Could you check a few things on this model? Use its own coordinates, in mm. A direction names the side the tool comes from. Give positions to 0.01 mm unless a question says otherwise; leave off trailing zeros. Write each loop counter-clockwise with the first axis right and the second up, starting at its lowest first coordinate (ties: lowest second). Pieces come first, ordered by that corner, then holes. Notation, with made-up numbers: (31.25, 20.25) - (44.25, 20.25) arc R27 cw to (44.25, 39.25) - close; hole circle Ø1 at (57.5, 69). An arc over 180 degrees is marked (long way). Answer in a Markdown table with one row per item.
from build123d import *

# Parameters (mm, degrees)
ESQUISSE1_W        = 155
ESQUISSE1_H        = 34
BOSS_EXTRU_1_DEPTH = 49
ESQUISSE2_R        = 2
BOSS_EXTRU_2_DEPTH = 5


with BuildPart() as part:
    # Esquisse1 → Boss.-Extru.1 (new body)
    with BuildSketch(Plane(origin=(0, 0, 0), x_dir=(1, 0, 0), z_dir=(0, 1, 0))):
        with Locations((77.5, 17)):
            Rectangle(ESQUISSE1_W, ESQUISSE1_H)
    extrude(amount=BOSS_EXTRU_1_DEPTH)

    # Esquisse2 → Boss.-Extru.2 (add)
    with BuildSketch(Plane(origin=(155, 0, 0), x_dir=(0, 0, -1), z_dir=(1, 0, 0))):
        with Locations(Location((14.5, 46, 0), (0, 0, 180))):
            Circle(ESQUISSE2_R)
        with Locations(Location((19.5, 46, 0), (0, 0, 180))):
            Circle(ESQUISSE2_R)
    extrude(amount=BOSS_EXTRU_2_DEPTH)


solid = part.part
1) Will this pin go through, and if not, where does the flat tip stop? P1, Ø8, axis at y = 39.5, z = -8, coming from the +X side.
Check values:
| item | result |
|---|---|
| P1 | stops at x = 155 |
2) If I drill on line 1 (X direction, y = 36, z = -13.5), over which ranges is the centre line in solid material (lowest first)?
Check values:
| item | result |
|---|---|
| line 1 | x = 0 to 155 |
3) On a 3-axis mill with a long thin cutter (end or side, diameter ignored), from which of +Z, -Z, +X, -X, +Y, -Y can I reach the whole of each face in a straight line? I mean faces 5 (the face through (0, 24, -17)), 6 (the face through (157.465, 47.952, -14.934)). Say none if no direction works.
Check values:
| item | result |
|---|---|
| face 5 | +Z, -Z, -X, +Y, -Y |
| face 6 | +X |
4) Imagine slicing it at C-C (y = 14). List the corners of the cut face in (x, z) for me.
Check values:
| item | result |
|---|---|
| outline | (0, -34) - (155, -34) - (155, 0) - (0, 0) - close |
5) Imagine slicing it at A-A (y = 46). List the corners of the cut face in (x, z) for me, then the cut area to 3 significant figures.
Check values:
| item | result |
|---|---|
| outline | (0, -34) - (155, -34) - (155, -21.5) - (160, -21.5) - (160, -17.5) - (155, -17.5) - (155, -16.5) - (160, -16.5) - (160, -12.5) - (155, -12.5) - (155, 0) - (0, 0) - close |
| area | 5,310 mm2 |
6) Imagine slicing it at D-D (z = -6.5). List the corners of the cut face in (x, y) for me.
Check values:
| item | result |
|---|---|
| outline | (0, 0) - (155, 0) - (155, 49) - (0, 49) - close |
7) Imagine slicing it at B-B (z = -19.5). List the corners of the cut face in (x, y) for me, then the cut area to 4 significant figures.
Check values:
| item | result |
|---|---|
| outline | (0, 0) - (155, 0) - (155, 44) - (160, 44) - (160, 48) - (155, 48) - (155, 49) - (0, 49) - close |
| area | 7,615 mm2 |
8) We'd pull the mould along Z, two halves only. Please class faces 1 (the face through (76, 24, -34)), 2 (the face through (157.465, 47.952, -19.934)), 3 (the face through (160, 46, -15)), 4 (the face through (76, 24, 0)): +Z half, -Z half, draft (parallel to the pull), parting line (faces both ways), or undercut.
Check values:
| item | result |
|---|---|
| face 1 | -Z half |
| face 2 | undercut |
| face 3 | draft |
| face 4 | +Z half |
